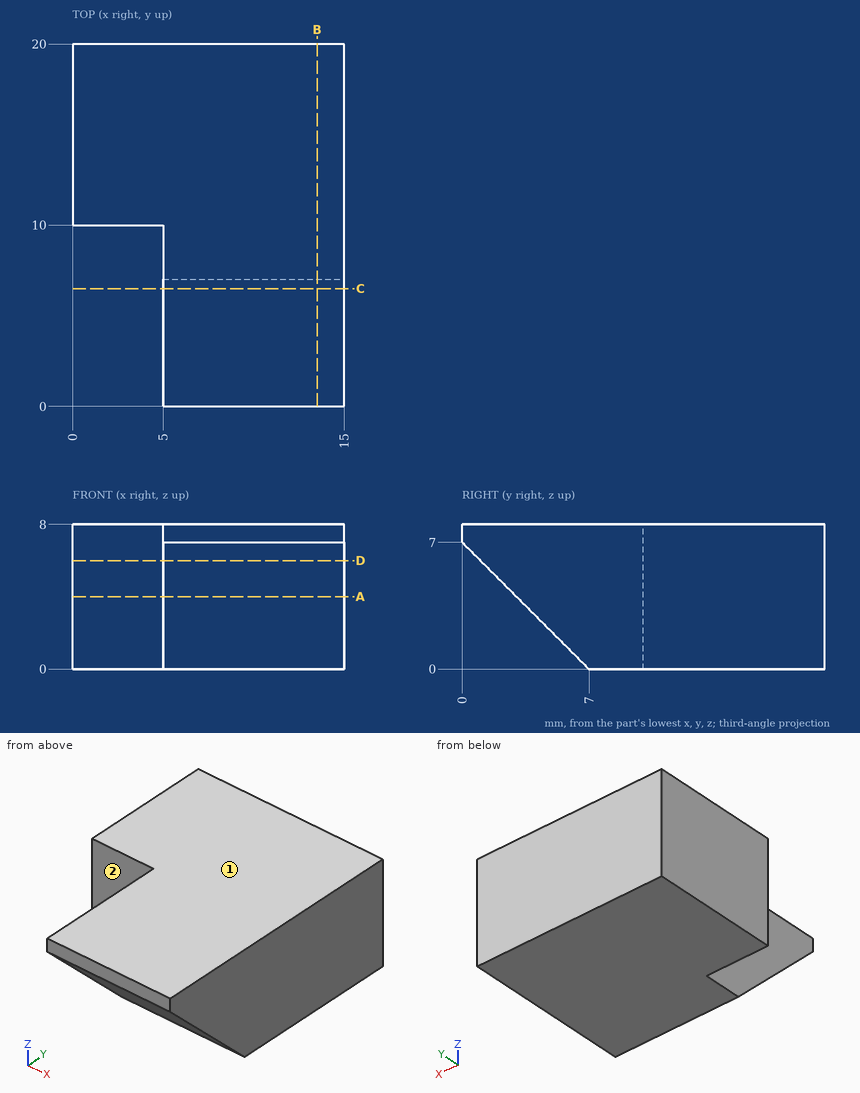
Geometry: see drawing. Coordinates: mm, zero at the bounding-box minimum. A direction names the side the tool comes from. Round coordinates to 2 decimals unless told otherwise and drop trailing zeros. Loops run counter-clockwise (first coordinate to the right, second up) from the corner with the lowest first, then second, coordinate; pieces in that order, holes last. Notation, with made-up numbers: M 65.25,49.25 L 117.25,49.25 A15 cw 117.25,67.25 Z; hole C 59.5,13 d9. An arc over 180 degrees is marked long. Use a Markdown table: item, result. Add a question column.
1. Cut plane A-A, the plane z = 4. Output: boundary loops of the cut face in (x, y), and give its area (3 significant figures).
2. Cut plane B-B, the plane x = 13.5. Output: boundary loops of the cut face in (y, z).
3. Ray query, line 1 along X through (y, z) = (2.25, 5); line 2 along Y through (x, z) = (4.25, 5); line 3 along Z through (x, y) = (12.25, 2.5). Return the intervals inside material, ascending. Write a range as [from, to].
4. Cut plane C-C, the plane y = 6.5. Output: boundary loops of the cut face in (x, z).
5. Set-up query: the marked faces 1 and 2. Return all of +Z, -Z, +X, -X, +Y, -Y with unobstructed straight access to the full face (end or side cutting, diameter ignored); none if empty.
6. Cut plane D-D, the plane z = 6. Output: boundary loops of the cut face in (x, y).
7. Contact query for flat-ended pins moving along their axis: pin 1 (1.5 mm diameter, centred on x = 8.5, y = 4.5, fed in from -Z); pin 2 (2.5 mm diameter, centred on x = 3, z = 3.5, fed in from -Y); pin 3 (2.5 mm diameter, centred on y = 5, z = 5.5, fed in from -X). Output: stop coordinate, or through.
Solution:
| question | item | result |
|---|---|---|
| 1 | outline | M 0,10 L 5,10 L 5,3 L 15,3 L 15,20 L 0,20 Z |
| 1 | area | 220 mm2 |
| 2 | outline | M 0,7 L 7,0 L 20,0 L 20,8 L 0,8 Z |
| 3 | line 1 | x = [5, 15] |
| 3 | line 2 | y = [10, 20] |
| 3 | line 3 | z = [4.5, 8] |
| 4 | outline | M 5,0.5 L 15,0.5 L 15,8 L 5,8 Z |
| 5 | face 1 | +Z, +X, -X, +Y, -Y |
| 5 | face 2 | +Z, -Z, -X, -Y |
| 6 | outline | M 0,10 L 5,10 L 5,1 L 15,1 L 15,20 L 0,20 Z |
| 7 | pin 1 | stops at z = 1.75 |
| 7 | pin 2 | stops at y = 10 |
| 7 | pin 3 | stops at x = 5 |
